Here's how the part is built. I have some questions about the finished solid (model axes, mm). A direction names the side the tool comes from. Round coordinates to 2 decimals unless told otherwise and drop trailing zeros. Loops run counter-clockwise (first coordinate to the right, second up) from the corner with the lowest first, then second, coordinate; pieces in that order, holes last. Notation, with made-up numbers: M 20,-22.5 L 39,-22.5 A25 cw 39,-5.5 Z; hole C 25,81.5 d1. An arc over 180 degrees is marked long. Use a Markdown table: item, result.
from build123d import *

# Parameters (mm, degrees)
F1_DEPTH  = 2
F2_R      = 1.9
F3_DEPTH  = 2.001
F5_W      = 19.2532
F5_H      = 15.0114
F6_DEPTH  = 2.001
F7_W      = 19.2532
F7_H      = 15.0114
F8_DEPTH  = 9.43
F9_W      = 11.43
F9_H      = 3.048
F10_DEPTH = 45.9292
F11_W     = 19.2532
F11_H     = 18.6114
F12_DEPTH = 1.778
F13_W     = 2.7532
F13_H     = 15.0114
F14_DEPTH = 2
F15_SIZE  = 1.8
F16_W     = 9
F16_H     = 11
F17_DEPTH = 2.001
F18_W     = 9
F18_H     = 11
F19_DEPTH = 4


# Not quite as in the source:
# - a fillet or chamfer that OpenCascade refuses, or shapes differently, is made with other operations: its cross-section is extruded or revolved along the edge and cut away or added


with BuildPart() as f1:
    # F0 (on Top) → F1 (new body)
    with BuildSketch(Plane.XY):
        with BuildLine():
            ThreePointArc((26.875, 8), (25.8498737342, 10.4748737342), (23.375, 11.5))
            Line((23.375, 11.5), (-23.375, 11.5))
            ThreePointArc((-23.375, 11.5), (-25.8498737342, 10.4748737342), (-26.875, 8))
            Line((-26.875, 8), (-26.875, -8))
            ThreePointArc((-26.875, -8), (-25.8498737342, -10.4748737342), (-23.375, -11.5))
            Line((-23.375, -11.5), (23.375, -11.5))
            ThreePointArc((23.375, -11.5), (25.8498737342, -10.4748737342), (26.875, -8))
            Line((26.875, -8), (26.875, 8))
        make_face()
    extrude(amount=F1_DEPTH)

    # F2 (on face) → F3 (cut, through all)
    with BuildSketch(Plane.XY.offset(2)):
        with Locations((-24, 0)):
            Circle(F2_R)
        with Locations((24, 0)):
            Circle(F2_R)
    extrude(amount=-F3_DEPTH, mode=Mode.SUBTRACT)

    # F4: chamfer of 1 on 2 edges, made by hand

    # F4_s1 → F4_t2 (revolve, cut)
    with BuildSketch(Plane.XZ):
        Polygon((-21.1, 0), (-22.1, 1), (-22.1, 0), align=None)
    revolve(axis=Axis((-24, 0, 0), (0, 0, 1)), mode=Mode.SUBTRACT)

    # F4_s3 → F4_t4 (revolve, cut)
    with BuildSketch(Plane.XZ):
        Polygon((26.9, 0), (25.9, 1), (25.9, 0), align=None)
    revolve(axis=Axis((24, 0, 0), (0, 0, 1)), mode=Mode.SUBTRACT)

    # F5 (on face) → F6 (cut, through all)
    with BuildSketch(Plane.XY.offset(2)):
        with Locations((-7.6266, 0)):
            Rectangle(F5_W, F5_H)
    extrude(amount=-F6_DEPTH, mode=Mode.SUBTRACT)

    # F7 (on face) → F8 (join)
    with BuildSketch(Plane.XY.offset(2)):
        with BuildLine():
            ThreePointArc((3.8, 8.0357), (3.4280256121, 8.9337256121), (2.53, 9.3057))
            Line((2.53, 9.3057), (-17.7832, 9.3057))
            ThreePointArc((-17.7832, 9.3057), (-18.6812256121, 8.9337256121), (-19.0532, 8.0357))
            Line((-19.0532, 8.0357), (-19.0532, -8.0357))
            ThreePointArc((-19.0532, -8.0357), (-18.6812256121, -8.9337256121), (-17.7832, -9.3057))
            Line((-17.7832, -9.3057), (2.53, -9.3057))
            ThreePointArc((2.53, -9.3057), (3.4280256121, -8.9337256121), (3.8, -8.0357))
            Line((3.8, -8.0357), (3.8, 8.0357))
        make_face()
        with Locations((-7.6266, 0)):
            Rectangle(F7_W, F7_H, mode=Mode.SUBTRACT)
    extrude(amount=F8_DEPTH)

    # F9 (on face) → F10 (cut, through all)
    with BuildSketch(Plane(origin=(-19.0532, 0, 0), x_dir=(0, -1, 0), z_dir=(-1, 0, 0))):
        with Locations((0, 7.366)):
            Rectangle(F9_W, F9_H)
    extrude(amount=-F10_DEPTH, mode=Mode.SUBTRACT)

    # F11 (on face) → F12 (cut)
    with BuildSketch(Plane.XY.offset(11.43)):
        with Locations((-7.6266, 0)):
            Rectangle(F11_W, F11_H)
    extrude(amount=-F12_DEPTH, mode=Mode.SUBTRACT)

    # F13 (on face) → F14 (join)
    with BuildSketch(Plane(origin=(0, 0, 0), x_dir=(1, 0, 0), z_dir=(0, 0, -1))):
        with Locations((0.6234, 0)):
            Rectangle(F13_W, F13_H)
    extrude(amount=-F14_DEPTH)

    # F15
    f15_edges = [f1.edges().sort_by_distance(p)[0] for p in [
        (-0.7532, 0, 2),
    ]]
    chamfer(f15_edges, length=F15_SIZE)

    # F16 (on face) → F17 (cut, through all)
    with BuildSketch(Plane.XY.offset(2)):
        with Locations((13, 0)):
            Rectangle(F16_W, F16_H)
    extrude(amount=-F17_DEPTH, mode=Mode.SUBTRACT)

    # F18 (on face) → F19 (join)
    with BuildSketch(Plane.XY.offset(2)):
        with BuildLine():
            ThreePointArc((18.03, -7.3), (18.9280256121, -6.9280256121), (19.3, -6.03))
            Line((19.3, -6.03), (19.3, 6.03))
            ThreePointArc((19.3, 6.03), (18.9280256121, 6.9280256121), (18.03, 7.3))
            Line((18.03, 7.3), (7.97, 7.3))
            ThreePointArc((7.97, 7.3), (7.0719743879, 6.9280256121), (6.7, 6.03))
            Line((6.7, 6.03), (6.7, -6.03))
            ThreePointArc((6.7, -6.03), (7.0719743879, -6.9280256121), (7.97, -7.3))
            Line((7.97, -7.3), (18.03, -7.3))
        make_face()
        with Locations((13, 0)):
            Rectangle(F18_W, F18_H, mode=Mode.SUBTRACT)
    extrude(amount=F19_DEPTH)


solid = f1.part
1. I need wall thicknesses on probe 1 along Y at (x, z) = (-1, 2.25); probe 2 along X at (y, z) = (2.25, 5.5); probe 3 along X at (y, z) = (7.25, 10). Which ranges of each line are inside material? Lowest first, please. Write a range as from..to.
Answer sheet:
| item | result |
|---|---|
| probe 1 | -9.31..-7.51, 7.51..9.31 |
| probe 2 | -19.05..-17.25, 2..3.8, 6.7..8.5, 17.5..19.3 |
| probe 3 | -19.05..-17.25, 2..3.8 |
2. Imagine slicing it at A-A, the plane z = 3.75. Write out the boundary of the cut face in (x, y).
Answer sheet:
| item | result |
|---|---|
| outline | M -19.05,-8.04 A1.27 ccw -17.78,-9.31 L 2.53,-9.31 A1.27 ccw 3.8,-8.04 L 3.8,8.04 A1.27 ccw 2.53,9.31 L -17.78,9.31 A1.27 ccw -19.05,8.04 Z; M 6.7,-6.03 A1.27 ccw 7.97,-7.3 L 18.03,-7.3 A1.27 ccw 19.3,-6.03 L 19.3,6.03 A1.27 ccw 18.03,7.3 L 7.97,7.3 A1.27 ccw 6.7,6.03 Z; hole M -17.25,-7.51 L 2,-7.51 L 2,7.51 L -17.25,7.51 Z; hole M 8.5,-5.5 L 17.5,-5.5 L 17.5,5.5 L 8.5,5.5 Z |
3. Imagine slicing it at C-C, the plane z = 8. Write out the boundary of the cut face in (x, y) (3 decimals), then the cut area to 3 significant figures.
Answer sheet:
| item | result |
|---|---|
| outline | M -19.053,-8.036 A1.27 ccw -17.783,-9.306 L 2.53,-9.306 A1.27 ccw 3.8,-8.036 L 3.8,-5.715 L 2,-5.715 L 2,-7.506 L -17.253,-7.506 L -17.253,-5.715 L -19.053,-5.715 Z; M -19.053,5.715 L -17.253,5.715 L -17.253,7.506 L 2,7.506 L 2,5.715 L 3.8,5.715 L 3.8,8.036 A1.27 ccw 2.53,9.306 L -17.783,9.306 A1.27 ccw -19.053,8.036 Z |
| area | 93.8 mm2 |
4. We'd pull the mould along X, two halves only. Please class faces 1 (the face through (2, 0, 5)), 2 (the face through (-18, -5.715, 7)), 3 (the face through (18.918, -6.938, 3.972)): +X half, -X half, draft (parallel to the pull), parting line (faces both ways), or undercut.
Answer sheet:
| item | result |
|---|---|
| face 1 | undercut |
| face 2 | draft |
| face 3 | +X half |
5. For pin 1 Ø3 at (x, z) = (14.5, 5.5) entering from -Y; pin 2 Ø3 at (y, z) = (3.5, 8.5) entering from -X; pin 3 Ø1.4 at (x, y) = (-11.5, -8) entering from +Z, each with a flat end and sliding along its axis, tell me the tip position at first contact or that it passes through.
Answer sheet:
| item | result |
|---|---|
| pin 1 | y = -7.3 |
| pin 2 | x = -19.05 |
| pin 3 | z = 9.65 |
6. Which directions (+Z, -Z, +X, -X, +Y, -Y) give clear straight access to the entire face, cutting with the end or side of a thin tool? Please do faces 4 (the face through (-18, 0, 5.842)), 5 (the face through (13, 5.5, 3)), 6 (the face through (3.8, -0.1, 5.6)).
Answer sheet:
| item | result |
|---|---|
| face 4 | -X |
| face 5 | +Z, -Z |
| face 6 | +Z, +Y, -Y |
7. Imagine slicing it at D-D, the plane x = 0. Write out the boundary of the cut face in (y, z), then the cut area to 3 significant figures.
Answer sheet:
| item | result |
|---|---|
| outline | M -11.5,0 L 11.5,0 L 11.5,2 L 9.31,2 L 9.31,9.65 L 7.51,9.65 L 7.51,0.95 L -7.51,0.95 L -7.51,9.65 L -9.31,9.65 L -9.31,2 L -11.5,2 Z |
| area | 57.8 mm2 |
8. Imagine slicing it at B-B, the plane x = 15.5. Write out the boundary of the cut face in (y, z).
Answer sheet:
| item | result |
|---|---|
| outline | M -11.5,0 L -5.5,0 L -5.5,6 L -7.3,6 L -7.3,2 L -11.5,2 Z; M 5.5,0 L 11.5,0 L 11.5,2 L 7.3,2 L 7.3,6 L 5.5,6 Z |
